Design review of the part built by this model. Coordinates are the model's own, in mm. Face numbers are marked on the shaded views. Give positions to 0.01 mm unless a question says otherwise; leave off trailing zeros. Write each loop counter-clockwise with the first axis right and the second up, starting at its lowest first coordinate (ties: lowest second). Pieces come first, ordered by that corner, then holes. Notation, with made-up numbers: M -8.5,85.25 L 40.5,85.25 A15 cw 40.5,106.25 Z; hole C 68.5,4.5 d1. An arc over 180 degrees is marked long. Answer in a Markdown table with one row per item.
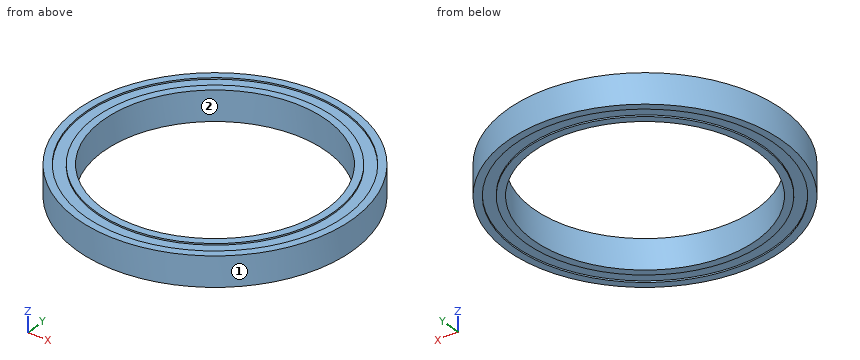
```python
from build123d import *


with BuildPart() as part:
    # 草图2 → 旋转1 (revolve)
    with BuildSketch(Plane(origin=(0, 0, 0), x_dir=(1, 0, 0), z_dir=(0, 1, 0))):
        Polygon((16, 2), (16, 1.8), (17.5, 1.8), (17.5, 2), (18.5, 2), (18.5, -2), (17.5, -2), (17.5, -1.8), (16, -1.8), (16, -2), (15, -2), (15, 2), align=None)
    revolve(axis=Axis((0, 0, 426.054329645), (0, 0, -1)))


solid = part.part
```
1) The part is to be moulded in two halves that separate along Y. For the marked faces 1 and 2, say which applies: released by +Y, released by -Y, zero draft, split by the parting line, or undercut.
Geometry says:
| item | result |
|---|---|
| face 1 | split by the parting line |
| face 2 | undercut |
2) To check wall thickness, follow probe 1 along Y at (x, z) = (0, -1.9); probe 2 along X at (y, z) = (0, -0.85). State the ranges of each line that lie inside material, in increasing order. Write a range as [from, to].
Geometry says:
| item | result |
|---|---|
| probe 1 | [-18.5, -17.5], [-16, -15], [15, 16], [17.5, 18.5] |
| probe 2 | [-18.5, -15], [15, 18.5] |
3) Add section C-C (z = -0.3). Write out the cut boundary in (x, y), and give its area (3 significant figures).
Geometry says:
| item | result |
|---|---|
| outline | C 0,0 d37; hole C 0,0 d30 |
| area | 368 mm^2 |
4) Add section A-A (x = 0). Write out the cut boundary in (y, z), and give its area (3 significant figures).
Geometry says:
| item | result |
|---|---|
| outline | M -18.5,-2 L -17.5,-2 L -17.5,-1.8 L -16,-1.8 L -16,-2 L -15,-2 L -15,2 L -16,2 L -16,1.8 L -17.5,1.8 L -17.5,2 L -18.5,2 Z; M 15,-2 L 16,-2 L 16,-1.8 L 17.5,-1.8 L 17.5,-2 L 18.5,-2 L 18.5,2 L 17.5,2 L 17.5,1.8 L 16,1.8 L 16,2 L 15,2 Z |
| area | 26.8 mm^2 |
5) Insertion check: P1, Ø2, axis at y = 8.5, z = 0, coming from the -X side; P2, Ø1.5, axis at x = -2, z = -1.5, coming from the +Y side; P3, Ø8, axis at x = -7, y = -0.5, coming from the -Z side; P4, Ø1, axis at y = 7, z = 0, coming from the +X side. Each pin has a flat end and moves straight along its axis. Give the tip position at first contact, or say it passes through.
Geometry says:
| item | result |
|---|---|
| P1 | x = -16.91 |
| P2 | y = 18.46 |
| P3 | through |
| P4 | x = 17.32 |
